CAD build for the part. Positions are in the model's coordinates, mm. A direction names the side the tool comes from. Give positions to 0.01 mm unless a question says otherwise; leave off trailing zeros. Loops run counter-clockwise (first coordinate to the right, second up) from the corner with the lowest first, then second, coordinate; pieces in that order, holes last. Notation, with made-up numbers: (32.25, 42) - (43.25, 42) arc R10 cw to (43.25, 56) - close; hole circle Ø7 at (-37, 77.25). An arc over 180 degrees is marked (long way). Return JSON: item names as keys, results as strings.
from build123d import *

# Parameters (mm, degrees)
F1_DEPTH = 63.5
F2_DEPTH = 7.9375
F3_DEPTH = 25.4
F5_R     = 6.35


# Not quite as in the source:
# - a feature names something its author has since deleted; it is built from what else it names


with BuildPart() as f1:
    # F0 (on Front) → F1 (new body, symmetric)
    with BuildSketch(Plane.XZ):
        Polygon((-41.275, 9.525), (-41.275, -9.525), (41.275, -9.525), (41.275, 9.525), (22.225, 9.525), align=None)
    extrude(amount=F1_DEPTH, both=True)

    # F0 (on Front) → F2 (join, symmetric)
    with BuildSketch(Plane.XZ):
        with BuildLine():
            add(Edge.make_bspline(
                [(-41.275, 9.525), (-41.112587778, 40.4556006324), (19.5290392467, 60.5257095831), (55.1792354288, 61.8695520445)],
                knots=[0, 0, 0, 0, 109.4601917253, 109.4601917253, 109.4601917253, 109.4601917253], degree=3))
            Line((-41.275, 9.525), (22.225, 9.525))
            Line((22.225, 9.525), (22.225, 27.0002))
            ThreePointArc((22.225, 27.0002), (31.7670866758, 50.9890168982), (55.1792354288, 61.8695520445))
        make_face()
    extrude(amount=F2_DEPTH, both=True)

    # F0 (on Front) → F3 (join, symmetric)
    with BuildSketch(Plane.XZ):
        with BuildLine():
            Line((22.225, 9.525), (41.275, 9.525))
            Line((41.275, 9.525), (41.275, 27.0002))
            ThreePointArc((41.275, 27.0002), (45.9246798487, 38.2255201513), (57.15, 42.8752))
            Line((57.15, 42.8752), (90.0369858318, 42.8752))
            Line((90.0369858318, 42.8752), (90.0369858318, 61.9252))
            Line((90.0369858318, 61.9252), (57.15, 61.9252))
            add(Edge.make_bspline(
                [(55.1792354288, 61.8695520445), (55.8450599549, 61.8946504554), (56.5021670835, 61.9132168549), (57.15, 61.9252)],
                knots=[109.4601917253, 109.4601917253, 109.4601917253, 109.4601917253, 111.5045361635, 111.5045361635, 111.5045361635, 111.5045361635], degree=3))
            ThreePointArc((55.1792354288, 61.8695520445), (31.7670866758, 50.9890168982), (22.225, 27.0002))
            Line((22.225, 27.0002), (22.225, 9.525))
        make_face()
    extrude(amount=F3_DEPTH, both=True)

    # F0 (on Front) → F4 (revolve)
    with BuildSketch(Plane.XZ):
        Polygon((90.0369858318, 68.1490233362), (90.0369858318, 61.9252), (90.0369858318, 42.8752), (90.0369858318, 39.5740233362), (115.4369858318, 39.5740233362), (115.4369858318, 68.1490233362), align=None)
    revolve(axis=Axis((90.0369858318, 0, 53.8615233362), (0, 0, -1)))

    # F5
    f5_edges = [f1.edges().sort_by_distance(p)[0] for p in [
        (-41.275, -63.5, 0),
        (41.275, -63.5, 0),
        (41.275, 63.5, 0),
        (-41.275, 63.5, 0),
    ]]
    fillet(f5_edges, radius=F5_R)


solid = f1.part
1. Drop flat-ended pins along their axis: P1, Ø5, axis at y = -19.5, z = 18, coming from the -X side (3 decimals); P2, Ø8, axis at y = 6, z = 24.5, coming from the -X side; P3, Ø15.5, axis at x = 63.5, z = 29.5, coming from the -Y side; P4, Ø15.5, axis at x = -13.5, z = 30.5, coming from the +Y side. Give the stop position or say it passes through.
Values follow:
{"P1": "stops at x = 22.225", "P2": "stops at x = -38.6", "P3": "passes through", "P4": "stops at y = 7.94"}
2. Pull direction X, two halves, no side cores. Call faces 1 (the face through (62, 0, 42.875)), 2 (the face through (22.225, 17, 18)), 3 (the face through (48, -25.4, 42)): +X half, -X half, draft (parallel to the pull), parting line (faces both ways), or undercut.
Values follow:
{"face 1": "undercut", "face 2": "-X half", "face 3": "draft"}
3. Drill centre lines: probe 1 along X at (y, z) = (-46, 9) (3 decimals); probe 2 along Y at (x, z) = (7, 38); probe 3 along Z at (x, y) = (-31, 36) (3 decimals). Where is each one in solid material? Low to high.
Values follow:
{"probe 1": "x = -41.275 to 41.275", "probe 2": "y = -7.94 to 7.94", "probe 3": "z = -9.525 to 9.525"}
4. Which spindle directions (+Z, -Z, +X, -X, +Y, -Y) get a long thin tool onto all of the face, cutting with end or side? Do faces 4 (the face through (22.225, -17, 18)), 5 (the face through (48, 25.4, 42)), 6 (the face through (63, 0, 61.925)). Say none if no direction does.
Values follow:
{"face 4": "+Z, -X, -Y", "face 5": "+Z, +X, -X, +Y", "face 6": "+Z, -X"}
5. Cut at A-A, the plane x = 79. Write the cut outline in (y, z).
Values follow:
{"outline": "(-25.4, 42.88) - (-22.88, 42.88) - (-22.88, 39.57) - (22.88, 39.57) - (22.88, 42.88) - (25.4, 42.88) - (25.4, 61.93) - (22.88, 61.93) - (22.88, 68.15) - (-22.88, 68.15) - (-22.88, 61.93) - (-25.4, 61.93) - close"}
6. Cut at B-B, the plane y = 53.5. Write the cut outline in (x, z) (3 decimals), plus the area to 3 significant figures.
Values follow:
{"outline": "(-41.275, -9.525) - (41.275, -9.525) - (41.275, 9.525) - (-41.275, 9.525) - close", "area": "1,570 mm²"}
7. Cut at C-C, the plane x = 62.5. Write the cut outline in (y, z), plus the area to 3 significant figures.
Values follow:
{"outline": "(-25.4, 42.88) - (25.4, 42.88) - (25.4, 61.93) - (-25.4, 61.93) - close", "area": "968 mm²"}
